Geometry check sheet. Reference: drawing and pictorial views, mm from the part's lowest x, y, z. A direction names the side the tool comes from. Coordinates: 2 decimals unless noted, no trailing zeros. Write each loop counter-clockwise with the first axis right and the second up, starting at its lowest first coordinate (ties: lowest second). Pieces come first, ordered by that corner, then holes. Notation, with made-up numbers: (38, 4) -> (77, 4) arc R21 cw to (77, 43) -> close; hole circle Ø4 at (52.5, -27). An arc over 180 degrees is marked (long way). Answer in a Markdown table with one row per item.
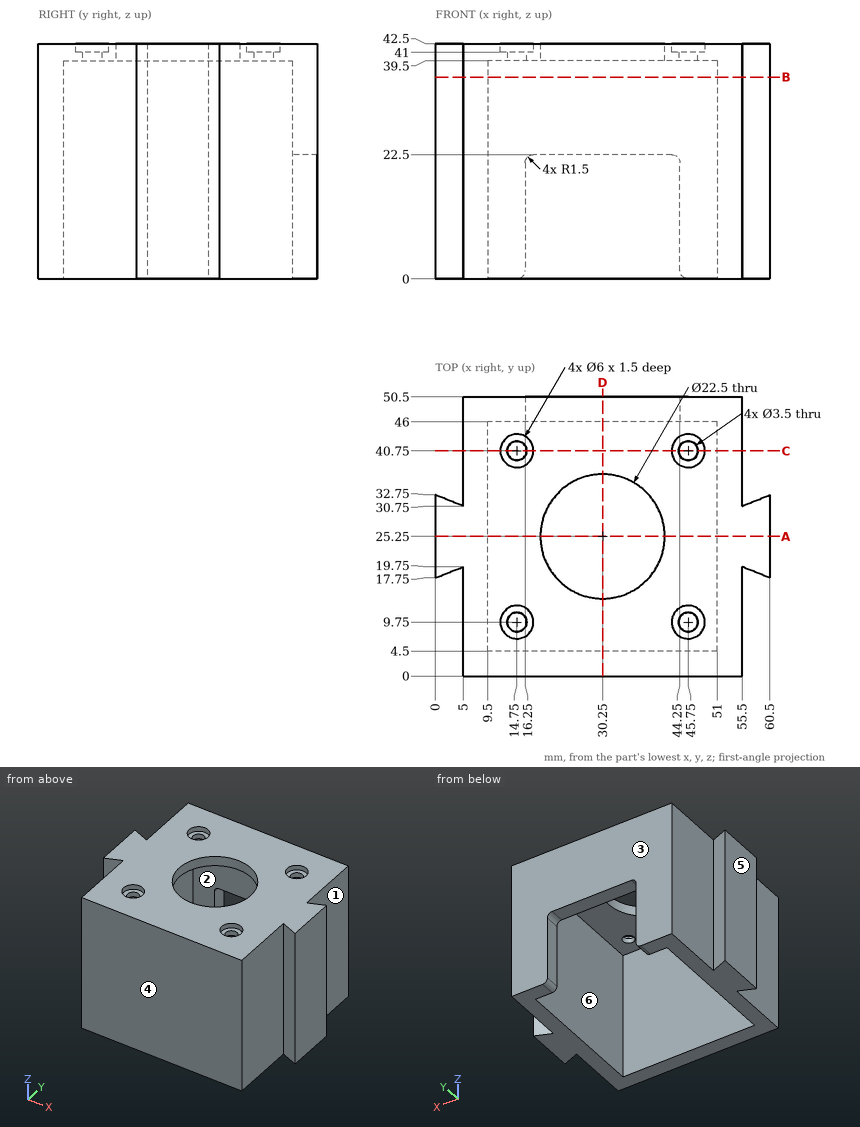
1. Thickness scan on line 1 (X direction, y = 40.75, z = 40.6); line 2 (Y direction, x = 30.25, z = 40.5); line 3 (X direction, y = 17, z = 4). Record the ranges inside material, lowest first. Write a range as from..to.
Geometry says:
| item | result |
|---|---|
| line 1 | 5..13, 16.5..44, 47.5..55.5 |
| line 2 | 0..14, 36.5..50.5 |
| line 3 | 5..9.5, 51..55.5 |
2. Mould release check, pull along Y, two halves, no side actions. Record for the marked faces 1, 2, 3 and 4: released by +Y, released by -Y, zero draft, split by the parting line, or undercut.
Geometry says:
| item | result |
|---|---|
| face 1 | zero draft |
| face 2 | undercut |
| face 3 | released by +Y |
| face 4 | released by -Y |
3. Section check A-A, the plane y = 25.25. Record the boundary of the cut face in (x, z), plus the area to 4 significant figures.
Geometry says:
| item | result |
|---|---|
| outline | (0, 0) -> (9.5, 0) -> (9.5, 39.5) -> (19, 39.5) -> (19, 42.5) -> (0, 42.5) -> close; (41.5, 39.5) -> (51, 39.5) -> (51, 0) -> (60.5, 0) -> (60.5, 42.5) -> (41.5, 42.5) -> close |
| area | 864.5 mm^2 |
4. Section check C-C, the plane y = 40.75. Record the boundary of the cut face in (x, z).
Geometry says:
| item | result |
|---|---|
| outline | (5, 0) -> (9.5, 0) -> (9.5, 39.5) -> (13, 39.5) -> (13, 41) -> (11.75, 41) -> (11.75, 42.5) -> (5, 42.5) -> close; (16.5, 39.5) -> (44, 39.5) -> (44, 41) -> (42.75, 41) -> (42.75, 42.5) -> (17.75, 42.5) -> (17.75, 41) -> (16.5, 41) -> close; (47.5, 39.5) -> (51, 39.5) -> (51, 0) -> (55.5, 0) -> (55.5, 42.5) -> (48.75, 42.5) -> (48.75, 41) -> (47.5, 41) -> close |
5. Depth check by flat-ended pin: P1, Ø3, axis at y = 42.5, z = 32, coming from the -X side; P2, Ø8, axis at x = 14.75, y = 40.75, coming from the +Z side; P3, Ø5, axis at x = 45.75, y = 9.75, coming from the +Z side; P4, Ø2, axis at y = 47.5, z = 14, coming from the +X side. Enter the tip coordinate at first touch or a pass-through.
Geometry says:
| item | result |
|---|---|
| P1 | x = 5 |
| P2 | z = 42.5 |
| P3 | z = 41 |
| P4 | x = 55.5 |
6. Section check B-B, the plane z = 36.5. Record the boundary of the cut face in (x, y), plus the area to 3 significant figures.
Geometry says:
| item | result |
|---|---|
| outline | (0, 17.75) -> (5, 19.75) -> (5, 0) -> (55.5, 0) -> (55.5, 19.75) -> (60.5, 17.75) -> (60.5, 32.75) -> (55.5, 30.75) -> (55.5, 50.5) -> (5, 50.5) -> (5, 30.75) -> (0, 32.75) -> close; hole (9.5, 4.5) -> (51, 4.5) -> (51, 46) -> (9.5, 46) -> close |
| area | 958 mm^2 |
7. Section check D-D, the plane x = 30.25. Record the boundary of the cut face in (y, z), plus the area to 3 significant figures.
Geometry says:
| item | result |
|---|---|
| outline | (0, 0) -> (4.5, 0) -> (4.5, 39.5) -> (14, 39.5) -> (14, 42.5) -> (0, 42.5) -> close; (36.5, 39.5) -> (46, 39.5) -> (46, 22.5) -> (50.5, 22.5) -> (50.5, 42.5) -> (36.5, 42.5) -> close |
| area | 338 mm^2 |
8. Tool access check on the marked faces 5 and 6. Record the directions out of +Z, -Z, +X, -X, +Y, -Y that give a thin tool (end or side, any length) a straight path to the whole face; none if there is none.
Geometry says:
| item | result |
|---|---|
| face 5 | +Z, -Z, -X, +Y, -Y |
| face 6 | -Z |
